Check sheet for the drawn part. Datum: minimum x, y, z corner. Units: mm. Round coordinates to 2 decimals unless told otherwise and drop trailing zeros. Write each loop counter-clockwise with the first axis right and the second up, starting at its lowest first coordinate (ties: lowest second). Pieces come first, ordered by that corner, then holes. Notation, with made-up numbers: (79, -36) - (118, -36) arc R19 ccw to (118, -32) - close; hole circle Ø8 at (-17, 56). An arc over 180 degrees is marked (long way). Answer as a JSON object with one key per item and string values.
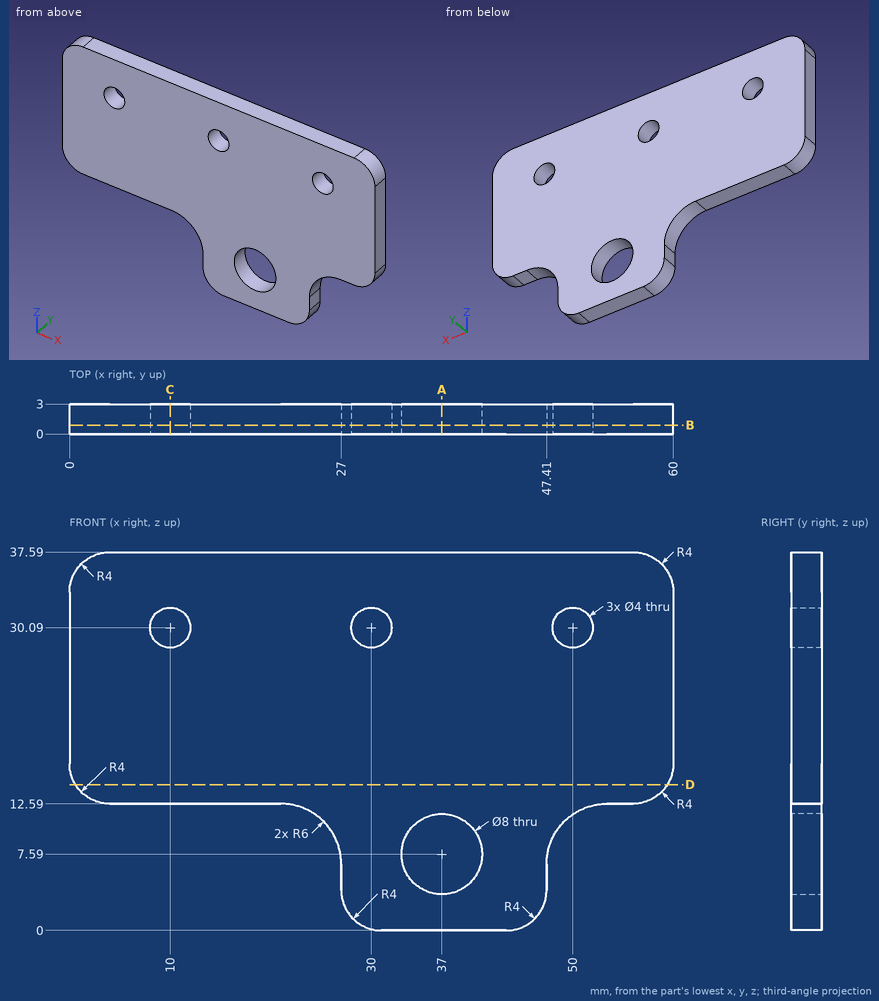
1. Cross-section at D-D (z = 14.5). Record the boundary of the cut face in (x, y).
Completed:
{"outline": "(0.59, 0) - (59.41, 0) - (59.41, 3) - (0.59, 3) - close"}
2. Go/stop test with a flat-tipped pin: pin 1 (1.3 mm diameter, centred on y = 2, z = 5, fed in from -X). Record where the tip stops, or that it passes through.
Completed:
{"pin 1": "stops at x = 27"}
3. Cross-section at A-A (x = 37). Record the boundary of the cut face in (y, z).
Completed:
{"outline": "(0, 0) - (3, 0) - (3, 3.59) - (0, 3.59) - close; (0, 11.59) - (3, 11.59) - (3, 37.59) - (0, 37.59) - close"}
4. Material ranges on probe 1 along X at (y, z) = (1.55, 31); probe 2 along Z at (x, y) = (13, 1.2); probe 3 along Z at (x, y) = (40, 2.4) (1 decimal), recorded low to high. Write a range as from..to.
Completed:
{"probe 1": "x = 0..8.22, 11.78..28.22, 31.78..48.22, 51.78..60", "probe 2": "z = 12.59..37.59", "probe 3": "z = 0..4.9, 10.2..37.6"}
5. Cross-section at B-B (y = 0.9). Record the boundary of the cut face in (x, z).
Completed:
{"outline": "(0, 16.59) arc R4 ccw to (4, 12.59) - (21, 12.59) arc R6 cw to (27, 6.59) - (27, 4) arc R4 ccw to (31, 0) - (43.41, 0) arc R4 ccw to (47.41, 4) - (47.41, 6.59) arc R6 cw to (53.41, 12.59) - (56, 12.59) arc R4 ccw to (60, 16.59) - (60, 33.59) arc R4 ccw to (56, 37.59) - (4, 37.59) arc R4 ccw to (0, 33.59) - close; hole circle Ø4 at (10, 30.09); hole circle Ø4 at (30, 30.09); hole circle Ø8 at (37, 7.59); hole circle Ø4 at (50, 30.09)"}
6. Cross-section at C-C (x = 10). Record the boundary of the cut face in (y, z), plus the area to 3 significant figures.
Completed:
{"outline": "(0, 12.59) - (3, 12.59) - (3, 28.09) - (0, 28.09) - close; (0, 32.09) - (3, 32.09) - (3, 37.59) - (0, 37.59) - close", "area": "63.0 mm^2"}
